Geometry: final body of the model. Coordinates: model frame, mm. Face numbers are marked on the shaded views. A direction names the side the tool comes from. Round coordinates to 2 decimals unless told otherwise and drop trailing zeros. Loops run counter-clockwise (first coordinate to the right, second up) from the corner with the lowest first, then second, coordinate; pieces in that order, holes last. Notation, with made-up numbers: (52, 65.25) - (69, 65.25) arc R17 cw to (69, 77.25) - close; hole circle Ø7 at (-22.5, 34.5). An arc over 180 degrees is marked (long way). Return JSON: item names as keys, results as strings. Group by question number.
1. First-contact query: pin 1 Ø1.5 at (y, z) = (25.5, 37) entering from +X; pin 2 Ø12.5 at (x, y) = (-25.5, -2.5) entering from +Z; pin 3 Ø2 at (x, y) = (13, 3.5) entering from +Z. Flat tips, straight axial feed; report the tip coordinate or a pass-through.
2. Material intervals for probe 1 along Y at (x, z) = (-58.5, 48.5); probe 2 along Z at (x, y) = (-43.5, -46.5); probe 3 along Y at (x, z) = (-31, 4.5), sorted ascending.
3. Draft query along Y for the marked faces 1, 2 and 3. Return one class per face: +Y half, -Y half, draft (parallel to the pull), parting line (faces both ways), or undercut.
4. Set-up query: the marked faces 4, 5 and 6. Return all of +Z, -Z, +X, -X, +Y, -Y with unobstructed straight access to the full face (end or side cutting, diameter ignored); none if empty.
5. Section A-A on x = -17. Return loops of the section in (y, z).
6. Section C-C on y = -2. Return loops of the section in (x, z).
7. Section B-B on y = -20. Return loops of the section in (x, z), and give its area (3 significant figures).
8. Section D-D on y = 44. Return loops of the section in (x, z), and give its area (3 significant figures).
from build123d import *

# Parameters (mm, degrees)
F0_W      = 113.2952198386
F0_H      = 106.3001342118
F1_DEPTH  = 50.8
F3_DEPTH  = 106.3011342118
F4_W      = 24.8478278518
F4_H      = 11.2919552803
F5_DEPTH  = 113.2962198386
F6_R      = 6.1575495423
F6_R_2    = 6.1008384399
F6_R_3    = 6.2250154244
F6_R_4    = 5.8180696171
F7_DEPTH  = 12.7
F9_DEPTH  = 17.78
F11_DEPTH = 10.16


with BuildPart() as f1:
    # F0 (on Top) → F1 (new body)
    with BuildSketch(Plane.XY):
        with Locations((-11.4009939134, -2.1379012614)):
            Rectangle(F0_W, F0_H)
    extrude(amount=F1_DEPTH)

    # F2 (on face) → F3 (cut, through all)
    with BuildSketch(Plane.XZ.offset(55.2879683673)):
        Polygon((0, 50.8), (45.2466160059, 0), (45.2466160059, 50.8), align=None)
    extrude(amount=-F3_DEPTH, mode=Mode.SUBTRACT)

    # F4 (on face) → F5 (cut, through all)
    with BuildSketch(Plane(origin=(-68.0486038327, 0, 0), x_dir=(0, -1, 0), z_dir=(-1, 0, 0))):
        with Locations((-1.490868628, 45.1540223598)):
            Rectangle(F4_W, F4_H)
    extrude(amount=-F5_DEPTH, mode=Mode.SUBTRACT)

    # F6 (on face) → F7 (cut)
    with BuildSketch(Plane(origin=(25.2307356453, 0, 22.4725473876), x_dir=(0, 1, 0), z_dir=(0.7467442801, 0, 0.6651112539))):
        with Locations((-23.4444309026, 15.2448490262)):
            Circle(F6_R)
        with Locations((-21.4417409152, -13.7552563101)):
            Circle(F6_R_2)
        with Locations((31.4639918506, 13.4591702372)):
            Circle(F6_R_3)
        with Locations((30.6235197932, -17.3407215625)):
            Circle(F6_R_4)
    extrude(amount=-F7_DEPTH, mode=Mode.SUBTRACT)

    # F8 (on face) → F9 (cut)
    with BuildSketch(Plane.XZ.offset(55.2879683673)):
        Polygon((15.1122735132, 33.832908044), (12.8093063831, 0), (45.2466160059, 0), align=None)
    extrude(amount=-F9_DEPTH, mode=Mode.SUBTRACT)

    # F10 (on face) → F11 (cut)
    with BuildSketch(Plane(origin=(0, 0, 0), x_dir=(1, 0, 0), z_dir=(0, 0, -1))):
        Polygon((-14.4420871511, 35.5851622298), (-14.4420871511, 55.2879683673), (-68.0486038327, 55.2879683673), (-68.0486038327, 42.1527642757), (-68.0486038327, 35.5851622298), align=None)
    extrude(amount=-F11_DEPTH, mode=Mode.SUBTRACT)


solid = f1.part
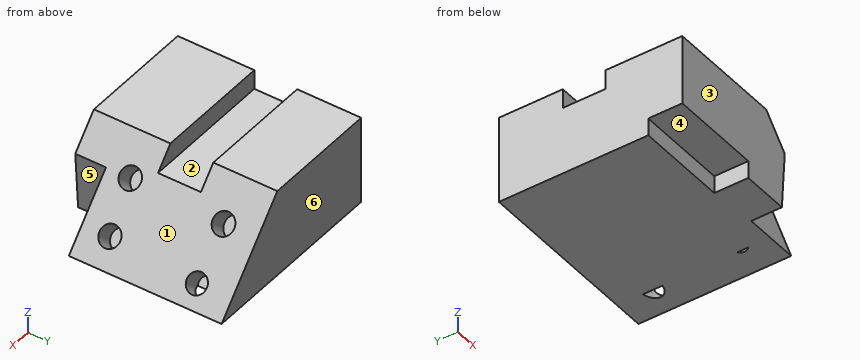
Taken from the geometry:
{
 "1": {"pin 1": "x = 12.96", "pin 2": "z = 39.51", "pin 3": "z = 37.33"},
 "2": {"probe 1": "-55.29 to -10.93, 13.91 to 51.01", "probe 2": "10.16 to 50.8", "probe 3": "-35.59 to 51.01"},
 "3": {"face 1": "draft", "face 2": "undercut", "face 3": "-Y half"},
 "4": {"face 4": "-Z, -X, -Y", "face 5": "-Z, +X, -Y", "face 6": "+Z, -Z, +X, -X, +Y"},
 "5": {"outline": "(-55.29, 10.16) - (-35.59, 10.16) - (-35.59, 0) - (51.01, 0) - (51.01, 50.8) - (13.91, 50.8) - (13.91, 39.51) - (-10.93, 39.51) - (-10.93, 50.8) - (-55.29, 50.8) - close"},
 "6": {"outline": "(-68.05, 0) - (45.25, 0) - (10.06, 39.51) - (-68.05, 39.51) - close"},
 "7": {"outline": "(-68.05, 0) - (28.24, 0) - (20.95, 8.18) - (30.44, 16.63) - (18.49, 30.05) - (9, 21.6) - (2.21, 29.22) - (11.7, 37.67) - (0, 50.8) - (-68.05, 50.8) - close; (29.59, 0) - (45.25, 0) - (38.32, 7.77) - close", "area": "4,330 mm2"},
 "8": {"outline": "(-68.05, 0) - (45.25, 0) - (0, 50.8) - (-68.05, 50.8) - close", "area": "4,610 mm2"}
}
